Here's how the part is built. I have some questions about the finished solid (model axes, mm). A direction names the side the tool comes from. Round coordinates to 2 decimals unless told otherwise and drop trailing zeros. Order: outer loops, then holes, each group sorted by start corner. A loop starts at its lowest first (then second) coordinate and runs counter-clockwise, first axis right, second up. Notation, with made-up numbers: M 16.5,56.5 L 38.5,56.5 A23 cw 38.5,72.5 Z; hole C 65.25,77.25 d5. An arc over 180 degrees is marked long. Use one line per item in the form item = value. Start each with the question number.
```python
from build123d import *

# Parameters (mm, degrees)
F0_R     = 39.751
F0_R_2   = 38.1
F1_DEPTH = 127
F2_R     = 47.625
F2_R_2   = 39.751
F3_DEPTH = 101.6
F4_R     = 7.62


with BuildPart() as f1:
    # F0 (on Front) → F1 (new body, symmetric)
    with BuildSketch(Plane.XZ):
        Circle(F0_R)
        Circle(F0_R_2, mode=Mode.SUBTRACT)
    extrude(amount=F1_DEPTH, both=True)

    # F2 (on Front) → F3 (join, symmetric)
    with BuildSketch(Plane.XZ):
        Circle(F2_R)
        Circle(F2_R_2, mode=Mode.SUBTRACT)
    extrude(amount=F3_DEPTH, both=True)

    # F4
    f4_edges = [f1.edges().sort_by_distance(p)[0] for p in [
        (-47.625, -101.6, 0),
        (-47.625, 101.6, 0),
    ]]
    fillet(f4_edges, radius=F4_R)


solid = f1.part
```
1) Will these pins go through, and if not, where does the flat tip stop? pin 1 Ø8 at (x, y) = (-32, 55.5) entering from +Z; pin 2 Ø12 at (x, y) = (-9, -95) entering from +Z; pin 3 Ø8 at (y, z) = (-46.5, -34.5) entering from +X.
2) If we mould it in two halves opening along Z, with no side actions, what happens to faces 1 (the cylindrical face through (-30.235, 1.778, -23.183)), 2 (the cylindrical face through (-8.617, 114.122, -38.806))? For each: +Z half, -Z half, draft (parallel to the pull), parting line (faces both ways), or undercut.
3) If we section it at A-A on z = 0: Write out the boundary of the cut face in (x, y) (3 decimals), then the cut area to 3 significant figures.
4) If we section it at B-B on x = 0: Write out the boundary of the cut face in (y, z) (3 decimals).
5) On a 3-axis mill with a long thin cutter (end or side, diameter ignored), from which of +Z, -Z, +X, -X, +Y, -Y can I reach the whole of each face in a straight line? I mean faces 3 (the cylindrical face through (-8.617, -114.478, -38.806)), 4 (the cylindrical face through (-37.794, -1.316, -28.979)). Say none if no direction works.
6) If we section it at C-C on y = -60: Write out the boundary of the cut face in (x, z) (3 decimals).
7) If I drill on line 1 (Z direction, x = -1, y = 57.5); line 2 (X direction, y = 102, z = 12); line 3 (X direction, y = -62, z = -12.5), over which ranges is the centre line in solid material (lowest first)?
Completed:
q1.pin_1 = 38.52
q1.pin_2 = 47.53
q1.pin_3 = 36.58
q2.face_1 = undercut
q2.face_2 = parting line
q3.outline = M -47.625,-93.98 A7.62 ccw -40.005,-101.6 L -39.751,-101.6 L -39.751,-127 L -38.1,-127 L -38.1,127 L -39.751,127 L -39.751,101.6 L -40.005,101.6 A7.62 ccw -47.625,93.98 Z; M 38.1,-127 L 39.751,-127 L 39.751,-101.6 L 40.005,-101.6 A7.62 ccw 47.625,-93.98 L 47.625,93.98 A7.62 ccw 40.005,101.6 L 39.751,101.6 L 39.751,127 L 38.1,127 Z
q3.area = 3,990 mm²
q4.outline = M -127,-39.751 L -101.6,-39.751 L -101.6,-40.005 A7.62 ccw -93.98,-47.625 L 93.98,-47.625 A7.62 ccw 101.6,-40.005 L 101.6,-39.751 L 127,-39.751 L 127,-38.1 L -127,-38.1 Z; M -127,38.1 L 127,38.1 L 127,39.751 L 101.6,39.751 L 101.6,40.005 A7.62 ccw 93.98,47.625 L -93.98,47.625 A7.62 ccw -101.6,40.005 L -101.6,39.751 L -127,39.751 Z
q5.face_3 = -Y
q5.face_4 = +Y, -Y
q6.outline = C 0,0 d95.25; hole C 0,0 d76.2
q7.line_1 = -47.61 to -38.09, 38.09 to 47.61
q7.line_2 = -37.9 to -36.16, 36.16 to 37.9
q7.line_3 = -45.96 to -35.99, 35.99 to 45.96
